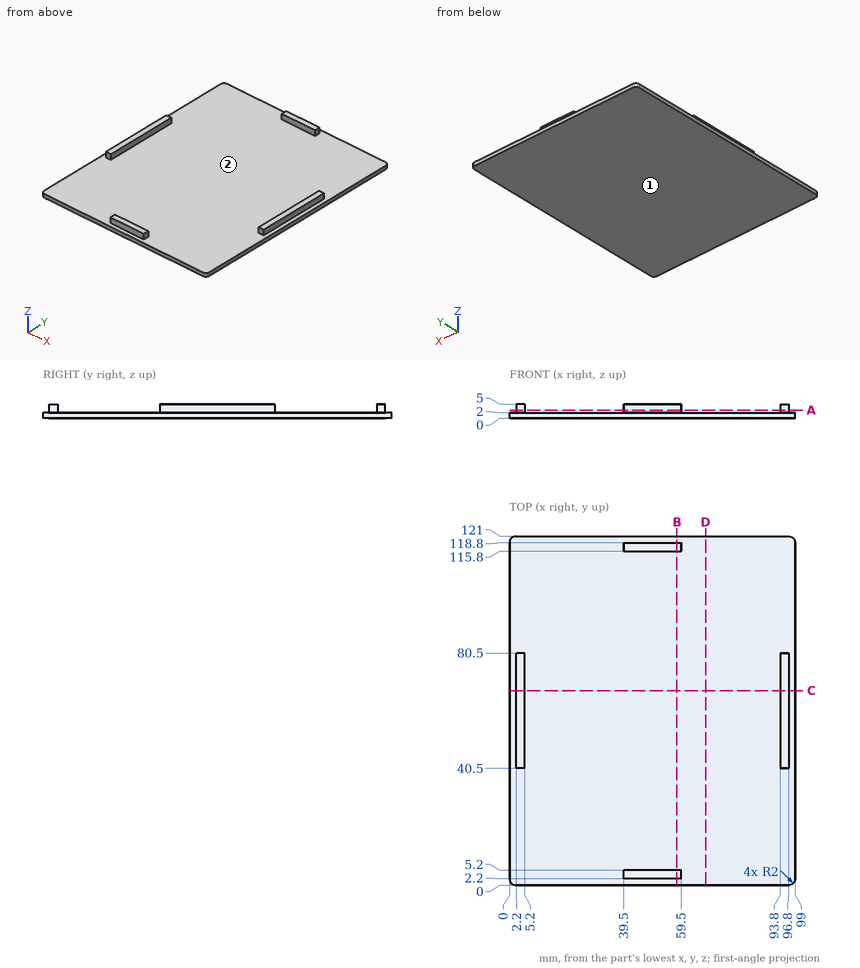
The figure shows three views and two pictorial views of one solid part (mm, origin at its lowest corner). Answer the questions. Coordinates: 2 decimals unless noted, no trailing zeros. Loops run counter-clockwise (first coordinate to the right, second up) from the corner with the lowest first, then second, coordinate; pieces in that order, holes last.
1) Find section D-D on x = 68. Write down the section's boundary in (y, z).
2) Find the intervals of material crossed by L1, parallel to X at y = 48, z = 4.2; L2, parallel to Y at x = 48.5, z = 3.1; L3, parallel to Z at x = 60, y = 58, in increasing order.
3) Find section B-B on x = 58. Write down the section's boundary in (y, z), then the cut area to 3 significant figures.
4) Determine the mould class of the marked faces 1 and 2 for opening direction X: pulls with the +X half, pulls with the -X half, needs draft (parallel to the pull), parting line crosses it, or undercut.
5) Flat-ended cylindrical pins translate along their axes: pin 1 Ø2.5 at (x, z) = (95, 3.5) entering from +Y; pin 2 Ø1.5 at (y, z) = (50.5, 3.5) entering from +X; pin 3 Ø1.5 at (y, z) = (3.5, 3) entering from +X. Find the tip coordinate at first contact, or state that the pin passes through.
6) Find section A-A on z = 2.9. Write down the section's boundary in (x, y).
7) Find section C-C on y = 67.5. Write down the section's boundary in (x, z).
Values:
1. outline: (0, 0) - (121, 0) - (121, 2) - (0, 2) - close
2. L1: x = 2.2 to 5.2, 93.8 to 96.8
2. L2: y = 2.2 to 5.2, 115.8 to 118.8
2. L3: z = 0 to 2
3. outline: (0, 0) - (121, 0) - (121, 2) - (118.8, 2) - (118.8, 5) - (115.8, 5) - (115.8, 2) - (5.2, 2) - (5.2, 5) - (2.2, 5) - (2.2, 2) - (0, 2) - close
3. area: 260 mm2
4. face 1: needs draft
4. face 2: undercut
5. pin 1: stops at y = 80.5
5. pin 2: stops at x = 96.8
5. pin 3: stops at x = 59.5
6. outline: (2.2, 40.5) - (5.2, 40.5) - (5.2, 80.5) - (2.2, 80.5) - close; (39.5, 2.2) - (59.5, 2.2) - (59.5, 5.2) - (39.5, 5.2) - close; (39.5, 115.8) - (59.5, 115.8) - (59.5, 118.8) - (39.5, 118.8) - close; (93.8, 40.5) - (96.8, 40.5) - (96.8, 80.5) - (93.8, 80.5) - close
7. outline: (0, 0) - (99, 0) - (99, 2) - (96.8, 2) - (96.8, 5) - (93.8, 5) - (93.8, 2) - (5.2, 2) - (5.2, 5) - (2.2, 5) - (2.2, 2) - (0, 2) - close
